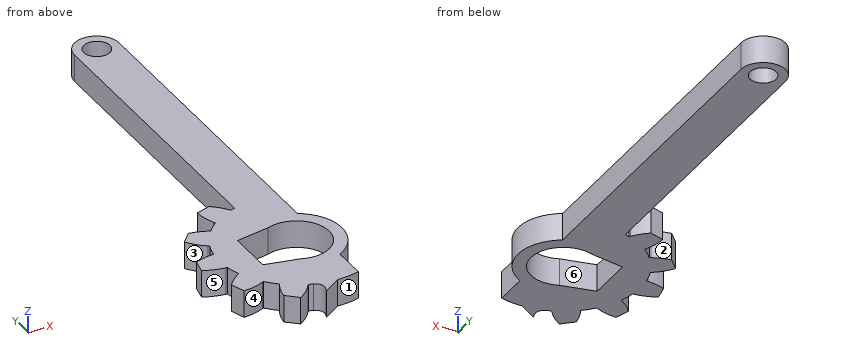
```python
from build123d import *

# Parameters (mm, degrees)
SKETCH1_R           = 1.45
BOSS_EXTRUDE1_DEPTH = 3
CUT_EXTRUDE2_DEPTH  = 46.173463436
SKETCH5_W           = 3.6
SKETCH5_H           = 3
FILLET1_R           = 1


with BuildPart() as part:
    # Sketch1 → Boss-Extrude1 (new body)
    with BuildSketch(Plane.XY.offset(1.9)):
        with BuildLine():
            Line((2.45, -8.139256723), (2.45, -4.358612164))
            ThreePointArc((2.45, -4.358612164), (5, 0), (2.45, 4.358612164))
            Line((2.45, 4.358612164), (2.45, 41))
            ThreePointArc((2.45, 41), (0, 43.45), (-2.45, 41))
            Line((-2.45, 41), (-2.45, 8.139256723))
            ThreePointArc((-2.45, 8.139256723), (-2.710254715, 8.056334116), (-2.967710696, 7.965092167))
            Line((-2.967710696, 7.965092167), (-3.054167872, 8.093270203))
            ThreePointArc((-3.054167872, 8.093270203), (-4.342095244, 9.472160372), (-5.994566265, 10.382893341))
            ThreePointArc((-5.994566265, 10.382893341), (-6.032083889, 8.496444973), (-5.481893659, 6.691622066))
            Line((-5.481893659, 6.691622066), (-5.414116812, 6.552658937))
            ThreePointArc((-5.414116812, 6.552658937), (-6.01040764, 6.01040764), (-6.552658937, 5.414116812))
            Line((-6.552658937, 5.414116812), (-6.691622066, 5.481893659))
            ThreePointArc((-6.691622066, 5.481893659), (-8.496444973, 6.032083889), (-10.382893341, 5.994566265))
            ThreePointArc((-10.382893341, 5.994566265), (-9.472160372, 4.342095244), (-8.093270203, 3.054167872))
            Line((-8.093270203, 3.054167872), (-7.965092167, 2.967710696))
            ThreePointArc((-7.965092167, 2.967710696), (-8.210369523, 2.199961883), (-8.381827508, 1.41243323))
            Line((-8.381827508, 1.41243323), (-8.536061531, 1.401648136))
            ThreePointArc((-8.536061531, 1.401648136), (-10.374179133, 0.975715399), (-11.989132531, 0))
            ThreePointArc((-11.989132531, 0), (-10.374179133, -0.975715399), (-8.536061531, -1.401648136))
            Line((-8.536061531, -1.401648136), (-8.381827508, -1.41243323))
            ThreePointArc((-8.381827508, -1.41243323), (-8.210369523, -2.199961883), (-7.965092167, -2.967710696))
            Line((-7.965092167, -2.967710696), (-8.093270203, -3.054167872))
            ThreePointArc((-8.093270203, -3.054167872), (-9.472160372, -4.342095244), (-10.382893341, -5.994566265))
            ThreePointArc((-10.382893341, -5.994566265), (-8.496444973, -6.032083889), (-6.691622066, -5.481893659))
            Line((-6.691622066, -5.481893659), (-6.552658937, -5.414116812))
            ThreePointArc((-6.552658937, -5.414116812), (-6.01040764, -6.01040764), (-5.414116812, -6.552658937))
            Line((-5.414116812, -6.552658937), (-5.481893659, -6.691622066))
            ThreePointArc((-5.481893659, -6.691622066), (-6.032083889, -8.496444973), (-5.994566265, -10.382893341))
            ThreePointArc((-5.994566265, -10.382893341), (-4.342095244, -9.472160372), (-3.054167872, -8.093270203))
            Line((-3.054167872, -8.093270203), (-2.967710696, -7.965092167))
            ThreePointArc((-2.967710696, -7.965092167), (-2.212026244, -8.207127384), (-1.437064557, -8.377639611))
            Line((-1.437064557, -8.377639611), (-1.984198903, -9.839001099))
            Line((-1.984198903, -9.839001099), (-0.052960828, -8.499835007))
            ThreePointArc((-0.052960828, -8.499835007), (1.212003867, -8.413147249), (2.45, -8.139256723))
        make_face()
        with Locations((0, 41)):
            Circle(SKETCH1_R, mode=Mode.SUBTRACT)
    extrude(amount=-BOSS_EXTRUDE1_DEPTH)

    # Sketch4 → Cut-Extrude2 (cut, through all)
    with BuildSketch(Plane.XY.offset(1.9)):
        with BuildLine():
            Line((-5.102940329, -2.6), (-1.358771093, -3.333727811))
            ThreePointArc((-1.358771093, -3.333727811), (-3.6, 0), (-1.358771093, 3.333727811))
            Line((-1.358771093, 3.333727811), (-5.102940329, 2.6))
            Line((-5.102940329, 2.6), (-5.102940329, -2.6))
        make_face()
    extrude(amount=-CUT_EXTRUDE2_DEPTH, mode=Mode.SUBTRACT)

    # Sketch5 → Cut-Revolve1 (revolve, cut)
    with BuildSketch(Plane(origin=(0, 0, 0), x_dir=(1, 0, 0), z_dir=(0, 1, 0))):
        with Locations((1.8, -0.4)):
            Rectangle(SKETCH5_W, SKETCH5_H)
    revolve(axis=Axis((0, 0, -1.1), (0, 0, 1)), mode=Mode.SUBTRACT)

    # Chamfer1
    # the kernel refuses this chamfer: 1.996823512, 1.412365401 mm, written as the material it takes off along each edge
    with BuildSketch(Plane(origin=(-5.994566265, -10.382893341, 6.307600342), x_dir=(0.8971018613244867, 0.44182377754953556, 0), z_dir=(0, 0, -1)), Plane(origin=(-10.382893341, -5.994566265, 6.307600342), x_dir=(0.9978248904640776, -0.06592031530834441, 0), z_dir=(0, 0, -1)), Plane(origin=(-11.989132531, 0, 6.307600342), x_dir=(0.8311815460161395, -0.5560011129145519, 0), z_dir=(0, 0, -1)), Plane(origin=(-10.382893341, 5.994566265, 6.307600342), x_dir=(0.4418237775496057, -0.8971018613244522, 0), z_dir=(0, 0, -1)), Plane(origin=(-5.994566265, 10.382893341, 6.307600342), x_dir=(-0.06592031530837167, -0.9978248904640757, 0), z_dir=(0, 0, -1))) as chamfer1_piece_1:
        with BuildLine():
            Line((1.33889649, 0), (0.700148491, -1.556942978))
            ThreePointArc((0.700148491, -1.556942978), (0.305807457, -0.828670891), (0, 0))
            ThreePointArc((0, 0), (0.684607685, 0.037444556), (1.33889649, 0))
        make_face()
    extrude(amount=11.815200684, mode=Mode.SUBTRACT)

    # Fillet1
    fillet1_edges = [part.edges().sort_by_distance(p)[0] for p in [
        (-1.437064557, -8.377639611, 0.4),
    ]]
    fillet(fillet1_edges, radius=FILLET1_R)


solid = part.part
```
For this review, take the finished solid that the model builds, in its own axes (mm). Face numbers are marked on the shaded views. A direction names the side the tool comes from. Round coordinates to 2 decimals unless told otherwise and drop trailing zeros. Order: outer loops, then holes, each group sorted by start corner. A loop starts at its lowest first (then second) coordinate and runs counter-clockwise, first axis right, second up. Notation, with made-up numbers: (1, 73.5) -> (9, 73.5) arc R32 ccw to (9, 101.5) -> close; hole circle Ø2 at (-19, 34). An arc over 180 degrees is marked (long way). Use a Markdown table: item, result.
Item 1: Take a section at C-C (y = 39). State the section outline as (x, z) points.
Resolved:
| item | result |
|---|---|
| outline | (-2.45, -1.1) -> (2.45, -1.1) -> (2.45, 1.9) -> (-2.45, 1.9) -> close |
Item 2: For pin 1 (1.5 mm diameter, centred on x = 3, z = 0, fed in from +Y); pin 2 (1.5 mm diameter, centred on y = 21.5, z = 0, fed in from -X); pin 3 (2.5 mm diameter, centred on x = 0, y = 41, fed in from -Z); pin 4 (0.9 mm diameter, centred on y = -7, z = 0, fed in from +X), all flat-tipped, find the tip position at first contact; note any pin that passes through.
Resolved:
| item | result |
|---|---|
| pin 1 | stops at y = 41.97 |
| pin 2 | stops at x = -2.45 |
| pin 3 | passes through |
| pin 4 | stops at x = 2.45 |
Item 3: Machinability: for the marked faces 4, 5 and 6, which of the approach directions +Z, -Z, +X, -X, +Y, -Y give a long, thin tool a straight path to every point of the face, cutting with its end or side? Answer none if there is none.
Resolved:
| item | result |
|---|---|
| face 4 | +Z, -Z, -Y |
| face 5 | +Z, -Z, -X |
| face 6 | +Z, -Z |
Item 4: For line 1 along Y through (x, z) = (0, -0.5); line 2 along Y through (x, z) = (1.25, 0.75); line 3 along X through (y, z) = (0, -0.25), list the stretches that pass through material, from the lowest coordinate up. Write a range as [from, to].
Resolved:
| item | result |
|---|---|
| line 1 | y = [-8.5, -3.6], [3.6, 39.55], [42.45, 43.45] |
| line 2 | y = [-8.41, -3.38], [3.38, 40.27], [41.73, 43.11] |
| line 3 | x = [-10.73, -5.1], [3.6, 5] |
Item 5: Draft analysis for pull direction Y (two halves, no side actions). For the marked faces 1, 2 and 3, state which applies: +Y half, -Y half, draft (parallel to the pull), parting line (faces both ways), or undercut.
Resolved:
| item | result |
|---|---|
| face 1 | -Y half |
| face 2 | +Y half |
| face 3 | undercut |
Item 6: Take a section at A-A (y = 0). State the section outline as (x, z) points, plus the area to 3 significant figures.
Resolved:
| item | result |
|---|---|
| outline | (-10.73, -1.1) -> (-5.1, -1.1) -> (-5.1, 1.9) -> (-10.73, 1.9) -> close; (3.6, -1.1) -> (5, -1.1) -> (5, 1.9) -> (3.6, 1.9) -> close |
| area | 21.1 mm² |
Item 7: Take a section at B-B (z = 1.3). State how many separate pieces and enclosed holes the cut face has, plus the area to 3 significant figures.
Resolved:
| item | result |
|---|---|
| separate pieces | 1 |
| enclosed holes | 2 |
| area | 309 mm² |
